Can you work these out from the model? Positions are in its coordinate system, mm. A direction names the side the tool comes from. Round coordinates to 2 decimals unless told otherwise and drop trailing zeros. Loops run counter-clockwise (first coordinate to the right, second up) from the corner with the lowest first, then second, coordinate; pieces in that order, holes last. Notation, with made-up numbers: M 55,35.25 L 100,35.25 A12 cw 100,41.25 Z; hole C -24.75,53 d4. An arc over 180 degrees is marked long. Return JSON: item names as keys, results as strings.
Autodesk Inventor part; units mm, degrees
ref_plane "YZ Plane" through (0, 0, 0) normal (1, 0, 0) x (0, 1, 0)
ref_plane "XZ Plane" through (0, 0, 0) normal (0, 1, 0) x (-1, 0, 0)
ref_plane "XY Plane" through (0, 0, 0) normal (0, 0, 1) x (1, 0, 0)
sketch "Sketch1" plane through (0, 0, 0) normal (1, 0, 0) x (0, 1, 0)
  line L0 (-7.2949, 20.7328) -> (24.4551, 20.7328)
  line L1 (24.4551, 20.7328) -> (24.4551, -55.4672)
  line L2 (24.4551, -55.4672) -> (-7.2949, -55.4672)
  line L3 (-7.2949, -55.4672) -> (-7.2949, 20.7328)
  point P0 (0, 0)
  dimension "d0" = 31.75
  dimension "d1" = 76.2
extrude "Extrusion1" add sketch "Sketch1" along normal blind 12.7
sketch "Sketch2" plane through (12.7, 0, 0) normal (1, 0, 0) x (0, 0, -1)
  line L0 (-9.5129, 22.6408) -> (33.105, 22.6408)
  line L1 (33.105, 22.6408) -> (33.105, -4.5028)
  line L2 (33.105, -4.5028) -> (-9.5129, -4.5028)
  line L3 (-9.5129, -4.5028) -> (-9.5129, 22.6408)
  line L4 (35.8954, 12.8742) -> (52.5113, 12.8742)
  line L5 (52.5113, 12.8742) -> (52.5113, 6.9127)
  line L6 (52.5113, 6.9127) -> (35.8954, 6.9127)
  line L7 (35.8954, 6.9127) -> (35.8954, 12.8742)
  point P0 (0, 0)
extrude "Extrusion2" cut sketch "Sketch2" against normal blind 6.35
fillet "Fillet1" radius 1.27 2 edges at (9.525, 12.8742, -52.5113) (9.525, 6.9127, -52.5113)
sketch "Sketch3" plane through (6.35, 0, 0) normal (1, 0, 0) x (0, 0, -1)
  circle A0 centre (23.0847, 9.3227) radius 2.6025
  circle A1 centre (-4.0588, 9.3227) radius 0.761
  point P0 (0, 0)
extrude "Extrusion3" cut sketch "Sketch3" against normal blind 1.27 contours A1
extrude "Extrusion4" add sketch "Sketch3" along normal blind 10.795 contours A0
properties part number "7.2 part 1"
Q1. If I drill on line 1 along Y through (x, z) = (6.75, -4); line 2 along Y through (x, z) = (10.25, -46.5); line 3 along Z through (x, y) = (12.25, -2) (3 decimals), over which ranges is the centre line in solid material (lowest first)?
Results:
{"line 1": "y = -7.29 to -4.5, 22.64 to 24.46", "line 2": "y = -7.29 to 6.91, 12.87 to 24.46", "line 3": "z = -55.467 to -33.105, 9.513 to 20.733"}
Q2. I'm going to push flat-ended pins straight in: pin 1 Ø3 at (y, z) = (11, -43) entering from +X; pin 2 Ø2 at (x, y) = (14.5, 8) entering from +Z; pin 3 Ø0.8 at (y, z) = (9, 4) entering from +X. Where does each tip first touch, or does it pass through?
Results:
{"pin 1": "stops at x = 6.35", "pin 2": "stops at z = -20.5", "pin 3": "stops at x = 5.08"}
Q3. Suppose I cut it at B-B, the plane y = 14. Please give me the cut outline in (x, z) (3 decimals), plus the area to 3 significant figures.
Results:
{"outline": "M 0,-55.467 L 12.7,-55.467 L 12.7,-33.105 L 6.35,-33.105 L 6.35,9.513 L 12.7,9.513 L 12.7,20.733 L 0,20.733 Z", "area": "697 mm2"}
Q4. Suppose I cut it at A-A, the plane x = 10.25. Please give me the cut outline in (y, z) (1 decimal), plus the area to 3 significant figures.
Results:
{"outline": "M -7.3,-55.5 L 24.5,-55.5 L 24.5,20.7 L -7.3,20.7 Z; C 9.3,-23.1 d5.2; hole M -4.5,-33.1 L 22.6,-33.1 L 22.6,9.5 L -4.5,9.5 Z; hole M 6.9,-51.2 A1.3 ccw 8.2,-52.5 L 11.6,-52.5 A1.3 ccw 12.9,-51.2 L 12.9,-35.9 L 6.9,-35.9 Z", "area": "1,190 mm2"}
Q5. Suppose I cut it at C-C, the plane z = -15. Please give me the cut outline in (x, y), plus the area to 3 significant figures.
Results:
{"outline": "M 0,-7.29 L 12.7,-7.29 L 12.7,-4.5 L 6.35,-4.5 L 6.35,22.64 L 12.7,22.64 L 12.7,24.46 L 0,24.46 Z", "area": "231 mm2"}
Q6. Thinking about a two-plate mould opening in Y: for faces 1 (the flat face through (12.7, 5, -34)), 2 (the cylindrical face through (11.672, 8.541, -25.567)), 3 (the flat face through (6, -7.295, -18)), 4 (the flat face through (10, 10, -35.895)), which applies, pulls with the +Y half, pulls with the -Y half, needs draft (parallel to the pull), parting line crosses it, or undercut?
Results:
{"face 1": "needs draft", "face 2": "undercut", "face 3": "pulls with the -Y half", "face 4": "undercut"}
Q7. On a 3-axis mill with a long thin cutter (end or side, diameter ignored), from which of +Z, -Z, +X, -X, +Y, -Y can I reach the whole of each face in a straight line? I mean faces 5 (the flat face through (0, 8, -17)), 6 (the cylindrical face through (9.481, 7.295, -52.149)). Say none if no direction works.
Results:
{"face 5": "+Z, -Z, -X, +Y, -Y", "face 6": "+X"}
Q8. Suppose I cut it at D-D, the plane x = 13.5. Please give me the cut outline in (y, z) (1 decimal).
Results:
{"outline": "C 9.3,-23.1 d5.2"}
